Check sheet for the modelled part. Datum: model origin and axes. Units: mm. A direction names the side the tool comes from. Coordinates: 2 decimals unless noted, no trailing zeros. Order: outer loops, then holes, each group sorted by start corner. A loop starts at its lowest first (then second) coordinate and runs counter-clockwise, first axis right, second up.
from build123d import *

# Parameters (mm, degrees)
BOSS_EXTRUDE1_DEPTH = 114.3
FILLET2_R           = 25.4
SKETCH2_W           = 63.5
SKETCH2_H           = 50.8
CUT_EXTRUDE1_DEPTH  = 25.4


with BuildPart() as part:
    # Sketch1 → Boss-Extrude1 (new body)
    with BuildSketch(Plane(origin=(0, 0, 0), x_dir=(1, 0, 0), z_dir=(0, 1, 0))):
        Polygon((0, 0), (0, 1143.361543418), (50.8, 1397), (101.6, 1143.361543418), (101.6, 0), align=None)
    extrude(amount=BOSS_EXTRUDE1_DEPTH)

    # Fillet2
    fillet2_edges = [part.edges().sort_by_distance(p)[0] for p in [
        (50.8, 57.15, -1397),
    ]]
    fillet(fillet2_edges, radius=FILLET2_R)

    # Sketch2 → Cut-Extrude1 (cut)
    with BuildSketch(Plane(origin=(0, 114.3, 0), x_dir=(1, 0, 0), z_dir=(0, 1, 0))):
        with Locations((50.8, 946.074302167)):
            Rectangle(SKETCH2_W, SKETCH2_H)
        with Locations((50.8, 1018.046396499)):
            Rectangle(SKETCH2_W, SKETCH2_H)
        with Locations((50.8, 874.822900853)):
            Rectangle(SKETCH2_W, SKETCH2_H)
        with Locations((50.8, 789.781020197)):
            Rectangle(SKETCH2_W, SKETCH2_H)
        with Locations((53.306135385, 713.133095909)):
            Rectangle(SKETCH2_W, SKETCH2_H)
    extrude(amount=-CUT_EXTRUDE1_DEPTH, mode=Mode.SUBTRACT)


solid = part.part
(1) Cross-section at A-A (z = -800). Enter the section's corners in (x, y).
Filled in:
outline: (0, 0) - (101.6, 0) - (101.6, 114.3) - (82.55, 114.3) - (82.55, 88.9) - (19.05, 88.9) - (19.05, 114.3) - (0, 114.3) - close
(2) Go/stop test with flat-tipped pins: P1, Ø6, axis at x = 57.5, y = 100.5, coming from the -Z side; P2, Ø6, axis at x = 30, y = 27, coming from the -Z side. Record where each tip stops, or that it passes through.
Filled in:
P1: stops at z = -1292.79
P2: stops at z = -1285.78
(3) Cross-section at D-D (z = -1176.5). Enter the section's corners in (x, y).
Filled in:
outline: (6.64, 0) - (94.96, 0) - (94.96, 114.3) - (6.64, 114.3) - close
(4) Release check for a two-part mould opening along X. For faces 1 (the flat face through (12.766, 56.35, -1207.101)), 2 (the flat face through (52, 0, -656)), 3 (the flat face through (53, 88.9, -713)) record: +X half, -X half, draft (parallel to the pull), parting line (faces both ways), or undercut.
Filled in:
face 1: -X half
face 2: draft
face 3: undercut
(5) Thickness scan on probe 1 along Z at (x, y) = (31.5, 106.5); probe 2 along Z at (x, y) = (54, 39); probe 3 along Y at (x, z) = (53, -896). Record the ranges inside material, lowest first.
Filled in:
probe 1: z = -1284.17 to -1043.45, -992.65 to -971.47, -920.67 to -900.22, -849.42 to -815.18, -764.38 to -738.53, -687.73 to 0
probe 2: z = -1292.86 to 0
probe 3: y = 0 to 88.9
(6) Tool access check on faces 4 (the flat face through (50, 102, -971.474)), 5 (the flat face through (101.6, 56, -580)). Record the directions out of +Z, -Z, +X, -X, +Y, -Y that give a thin tool (end or side, any length) a straight path to the whole face; none if there is none.
Filled in:
face 4: +Y
face 5: +Z, -Z, +X, +Y, -Y
(7) Cross-section at C-C (x = 65). Enter the section's corners in (y, z).
Filled in:
outline: (0, -1288.72) - (114.3, -1288.72) - (114.3, -1043.45) - (88.9, -1043.45) - (88.9, -992.65) - (114.3, -992.65) - (114.3, -971.47) - (88.9, -971.47) - (88.9, -920.67) - (114.3, -920.67) - (114.3, -900.22) - (88.9, -900.22) - (88.9, -849.42) - (114.3, -849.42) - (114.3, -815.18) - (88.9, -815.18) - (88.9, -764.38) - (114.3, -764.38) - (114.3, -738.53) - (88.9, -738.53) - (88.9, -687.73) - (114.3, -687.73) - (114.3, 0) - (0, 0) - close
(8) Cross-section at B-B (y = 53). Enter the section's corners in (x, z).
Filled in:
outline: (0, -1143.36) - (25.89, -1272.65) arc R25.4 ccw to (75.71, -1272.65) - (101.6, -1143.36) - (101.6, 0) - (0, 0) - close
